Part model, mm, in its own coordinate system. A direction names the side the tool comes from. Round coordinates to 2 decimals unless told otherwise and drop trailing zeros. Loops run counter-clockwise (first coordinate to the right, second up) from the corner with the lowest first, then second, coordinate; pieces in that order, holes last. Notation, with made-up numbers: (-14.5, -6) - (26.5, -6) arc R11 ccw to (26.5, 9) - close; hole circle Ø2 at (72.5, -30.5). An arc over 180 degrees is marked (long way). Write each question's results on one line, items separated by ' | '. Start each with the question number.
(1) Cut at A-A, the plane z = 75. List the corners of the cut face in (x, y).
(2) Flat gauge pins, fed straight in: P1, Ø1, axis at x = 8, y = 1.5, coming from the -Z side; P2, Ø1.2, axis at x = -4, z = 14.5, coming from the -Y side; P3, Ø1.1, axis at y = 1.5, z = 3.5, coming from the +X side. Where does each tip first touch, or does it go through?
(3) Drill centre lines: L1, parallel to X at y = 1.75, z = -10; L2, parallel to Z at x = -6.75, y = 0.65; L3, parallel to X at y = 0.45, z = 15. Where is each one in solid material? Low to high.
(4) Mould opens along Z. For faces 4 (the face through (-14.5, 1.5, -10)), 5 (the face through (-3, 0, 34)), 6 (the face through (-6.2, 0.7, 16.6)), 7 (the face through (-12, 1, 57)) say: released by +Z, released by -Z, zero draft, split by the parting line, or undercut.
(5) Cut at D-D, the plane x = 8.25. List the corners of the cut face in (y, z), then the cut area to 3 significant figures.
(6) Tool access for faces 1 (the face through (1, 1.5, 39)), 2 (the face through (-4, 1, 89)), 3 (the face through (-3, 3, 34)): list every direction of +Z, -Z, +X, -X, +Y, -Y with a clear straight run to the whole face (end or side of a thin tool).
(7) Cut at C-C, the plane z = 38. List the corners of the cut face in (x, y), then the cut area to 3 significant figures.
(8) Cut at B-B, the plane x = -13. List the corners of the cut face in (y, z).
from build123d import *

# Parameters (mm, degrees)
SKETCH_2_R          = 3
EXTRUDE_1_DEPTH     = 3
SKETCH_3_R          = 3.5
EXTRUDE_2_DEPTH     = 3
SKETCH_4_R          = 3.5
EXTRUDE_3_DEPTH     = 3
CUT_EXTRUDE_1_DEPTH = 107.618473768
CUT_EXTRUDE_2_DEPTH = 107.618473768
EXTRUDE_4_DEPTH     = 3
SKETCH_6_R          = 1.25
CUT_EXTRUDE_3_DEPTH = 107.618473768
SKETCH_6_3_R        = 2
SKETCH_6_3_R_2      = 1.25
CUT_EXTRUDE_4_DEPTH = 1.5


with BuildPart() as part:
    # Sketch 2 → Extrude 1 (new body)
    with BuildSketch(Plane(origin=(0, 0, 0), x_dir=(1, 0, 0), z_dir=(0, 1, 0))):
        with BuildLine():
            Line((-8, 0), (-15.238247957, -15.382059892))
            Line((-15.238247957, -15.382059892), (-8.643699882, -100.125861646))
            Line((-8.643699882, -100.125861646), (-8.61301011, -100.126871188))
            ThreePointArc((-8.61301011, -100.126871188), (-3.780099648, -105.28855468), (1.381583844, -100.455644218))
            Line((1.381583844, -100.455644218), (1.399355455, -100.456228817))
            Line((1.399355455, -100.456228817), (10.979274058, -19.016660498))
            Line((10.979274058, -19.016660498), (1.010362938, -1.749999943))
            ThreePointArc((1.010362938, -1.749999943), (-0.270725971, -0.46891107), (-2.020725942, 0))
            Line((-2.020725942, 0), (-8, 0))
        make_face()
        with Locations(Location((-3.615713133, -100.291257703, 0), (0, 0, 270))):
            Circle(SKETCH_2_R, mode=Mode.SUBTRACT)
        with BuildLine():
            ThreePointArc((-3.020725942, -2.381966011), (-0.520725942, -3.5), (-3.020725942, -4.618033989))
            Line((-3.020725942, -4.618033989), (-3.020725942, -2.381966011))
        make_face(mode=Mode.SUBTRACT)
        with Locations(Location((1.451061426, -22.124978573, 0), (0, 0, 270))):
            Circle(SKETCH_2_R, mode=Mode.SUBTRACT)
    extrude(amount=EXTRUDE_1_DEPTH)

    # Sketch 4 → Extrude 3 (add)
    with BuildSketch(Plane.XZ):
        with Locations((-5, 89)):
            Circle(SKETCH_4_R)
    extrude(amount=-EXTRUDE_3_DEPTH)

    # Sketch 4_3 → Cut-Extrude 1 (cut, through all)
    with BuildSketch(Plane.XZ):
        with BuildLine():
            ThreePointArc((-3.5, 89), (-3.60795306, 89.55875336), (-3.916273757, 90.037081207))
            Line((-3.916273757, 90.037081207), (-4.089754437, 87.807752956))
            ThreePointArc((-4.089754437, 87.807752956), (-3.655498541, 88.334931712), (-3.5, 89))
        make_face()
        with BuildLine():
            Line((-4.089754437, 87.807752956), (-3.916273757, 90.037081207))
            ThreePointArc((-3.916273757, 90.037081207), (-6.495478854, 89.116374378), (-4.089754437, 87.807752956))
        make_face()
    extrude(amount=-CUT_EXTRUDE_1_DEPTH, mode=Mode.SUBTRACT)

    # Sketch 4_4 → Cut-Extrude 2 (cut, through all)
    with BuildSketch(Plane.XZ):
        with BuildLine():
            ThreePointArc((1.384286867, 100.291257703), (1.127703357, 98.710118873), (0.384286867, 97.291257703))
            Line((0.384286867, 97.291257703), (10.979274058, 19.016660498))
            Line((10.979274058, 19.016660498), (1.399355455, 100.456228817))
            Line((1.399355455, 100.456228817), (1.381583844, 100.455644218))
            ThreePointArc((1.381583844, 100.455644218), (1.383611066, 100.373462071), (1.384286867, 100.291257703))
        make_face()
    extrude(amount=-CUT_EXTRUDE_2_DEPTH, mode=Mode.SUBTRACT)



with BuildPart() as body_2:
    # Sketch 3 → Extrude 2 (new body)
    with BuildSketch(Plane.XZ):
        with Locations(Location((-13, -10, 0), (0, 0, 270))):
            Circle(SKETCH_3_R)
        with BuildLine():
            Line((-12, -8.881966011), (-12, -11.118033989))
            ThreePointArc((-12, -11.118033989), (-14.5, -10), (-12, -8.881966011))
        make_face(mode=Mode.SUBTRACT)
    extrude(amount=-EXTRUDE_2_DEPTH)


with BuildPart() as part_1:
    add(part.part)

    add(body_2.part)  # Extrude 4 merges body 2
    # Sketch 5 → Extrude 4 (add)
    with BuildSketch(Plane.XZ):
        with BuildLine():
            Line((-10.28463728, -12.208348998), (0.694636778, 1.291651002))
            Line((0.694636778, 1.291651002), (-8, 0))
            Line((-8, 0), (-15.238247957, 15.382059892))
            Line((-15.238247957, 15.382059892), (-16.495653764, -9.825630381))
            ThreePointArc((-16.495653764, -9.825630381), (-11.746385015, -6.732210308), (-10.28463728, -12.208348998))
        make_face()
        with BuildLine():
            Line((-4, 90.118033989), (-4, 87.881966011))
            ThreePointArc((-4, 87.881966011), (-3.5, 89), (-4, 90.118033989))
        make_face()
    extrude(amount=-EXTRUDE_4_DEPTH)

    # Sketch 6 → Cut-Extrude 3 (cut, through all)
    with BuildSketch(Plane.XZ):
        with Locations(Location((-5, 15, 0), (0, 0, 270))):
            Circle(SKETCH_6_R)
        with Locations(Location((2, 38, 0), (0, 0, 270))):
            Circle(SKETCH_6_R)
        with Locations(Location((-5, 75, 0), (0, 0, 270))):
            Circle(SKETCH_6_R)
    extrude(amount=-CUT_EXTRUDE_3_DEPTH, mode=Mode.SUBTRACT)

    # Sketch 6_3 → Cut-Extrude 4 (cut)
    # profile 1 of 3: a face of its own
    with BuildSketch(Plane.XZ):
        with Locations(Location((-5, 15, 0), (0, 0, 270))):
            Circle(SKETCH_6_3_R)
        with Locations(Location((-5, 15, 0), (0, 0, 270))):
            Circle(SKETCH_6_3_R_2, mode=Mode.SUBTRACT)
    # profile 2 of 3: a face of its own
    with BuildSketch(Plane.XZ):
        with Locations(Location((2, 38, 0), (0, 0, 270))):
            Circle(SKETCH_6_3_R)
        with Locations(Location((2, 38, 0), (0, 0, 270))):
            Circle(SKETCH_6_3_R_2, mode=Mode.SUBTRACT)
    # profile 3 of 3: a face of its own
    with BuildSketch(Plane.XZ):
        with Locations(Location((-5, 75, 0), (0, 0, 270))):
            Circle(SKETCH_6_3_R)
        with Locations(Location((-5, 75, 0), (0, 0, 270))):
            Circle(SKETCH_6_3_R_2, mode=Mode.SUBTRACT)
    extrude(amount=-CUT_EXTRUDE_4_DEPTH, mode=Mode.SUBTRACT)


solid = part_1.part
A:
1) outline: (-10.6, 0) - (-7, 0) - (-7, 1.5) - (-6.25, 1.5) - (-6.25, 3) - (-10.6, 3) - close; (-3.75, 1.5) - (-3, 1.5) - (-3, 0) - (3.4, 0) - (3.4, 3) - (-3.75, 3) - close
2) P1: z = 12.99 | P2: y = 1.5 | P3: x = 2.34
3) L1: -16.5 to -14.5, -12 to -8.49 | L2: -7.86 to 14.03, 15.97 to 74.03, 75.97 to 104.19 | L3: -15.26 to -7, -3 to 8.66
4) face 4: undercut | face 5: zero draft | face 6: undercut | face 7: released by +Z
5) outline: (0, 14.29) - (3, 14.29) - (3, 39.18) - (0, 39.18) - close | area: 74.7 mm2
6) face 1: -Y | face 2: +Y, -Y | face 3: +Z, -Z, +X, -X, +Y
7) outline: (-13.48, 0) - (0, 0) - (0, 1.5) - (0.75, 1.5) - (0.75, 3) - (-13.48, 3) - close; (3.25, 1.5) - (4, 1.5) - (4, 0) - (8.41, 0) - (8.41, 3) - (3.25, 3) - close | area: 55.9 mm2
8) outline: (0, -13.5) - (3, -13.5) - (3, -11.5) - (0, -11.5) - close; (0, -8.5) - (3, -8.5) - (3, 44.14) - (0, 44.14) - close
